```python
from build123d import *

# Parameters (mm, degrees)
SKETCH285_W     = 17
SKETCH285_H     = 21
PAD190_DEPTH    = 29
SKETCH281_W     = 13.1
SKETCH281_H     = 17
POCKET037_DEPTH = 25.7
SKETCH268_W     = 11.5
SKETCH268_H     = 1.2
SKETCH268_W_2   = 1.4
SKETCH268_H_2   = 2
POCKET039_DEPTH = 26.8
SKETCH271_R     = 0.6
POCKET041_DEPTH = 50
SKETCH278_W     = 0.6
SKETCH278_H     = 3
POCKET038_DEPTH = 2.5


with BuildPart() as part:
    # Sketch285 → Pad190 (new body)
    with BuildSketch(Plane.XZ):
        with Locations((1.5, 2)):
            Rectangle(SKETCH285_W, SKETCH285_H)
    extrude(amount=PAD190_DEPTH)

    # Sketch281 (on Face5 of Pad190) → Pocket037 (cut)
    with BuildSketch(Plane(origin=(0, 0, 0), x_dir=(1, 0, 0), z_dir=(0, 1, 0))):
        with Locations((2.05, -2)):
            Rectangle(SKETCH281_W, SKETCH281_H)
    extrude(amount=-POCKET037_DEPTH, mode=Mode.SUBTRACT)

    # Sketch268 (on Face4 of Pocket037) → Pocket039 (cut)
    with BuildSketch(Plane(origin=(0, 0, 0), x_dir=(1, 0, 0), z_dir=(0, 1, 0))):
        Rectangle(SKETCH268_W, SKETCH268_H)
        with Locations((9.3, -6)):
            Rectangle(SKETCH268_W_2, SKETCH268_H_2)
    extrude(amount=-POCKET039_DEPTH, mode=Mode.SUBTRACT)

    # Sketch271 (on Face6 of Pocket039) → Pocket041 (cut)
    with BuildSketch(Plane(origin=(0, 0, -8.5), x_dir=(1, 0, 0), z_dir=(0, 0, -1))):
        with Locations((0, 2)):
            Circle(SKETCH271_R)
    extrude(amount=-POCKET041_DEPTH, mode=Mode.SUBTRACT)

    # Sketch278 (on Face21 of Pocket041) → Pocket038 (cut)
    with BuildSketch(Plane(origin=(8.6, 0, 0), x_dir=(0, 0, 1), z_dir=(1, 0, 0))):
        with Locations((0, -9)):
            Rectangle(SKETCH278_W, SKETCH278_H)
    extrude(amount=-POCKET038_DEPTH, mode=Mode.SUBTRACT)


solid = part.part
```
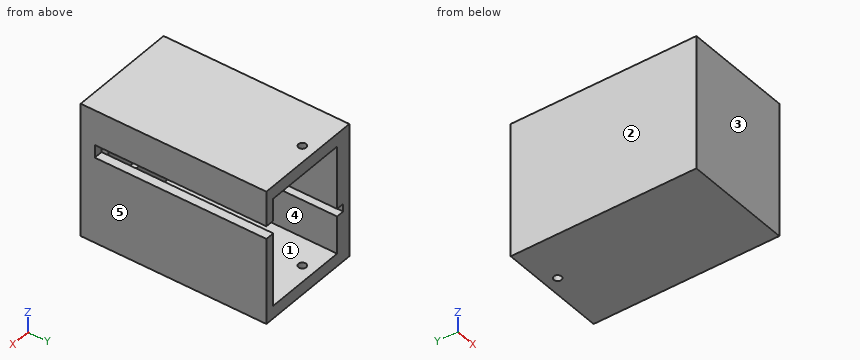
Read the model definition and answer for the solid it produces. Units are mm, in the model's axes. Face numbers are marked on the shaded views. A direction names the side the tool comes from. Coordinates: 2 decimals unless noted, no trailing zeros. Write each loop counter-clockwise with the first axis right and the second up, starting at its lowest first coordinate (ties: lowest second). Pieces come first, ordered by that corner, then holes. Notation, with made-up numbers: (19.25, -26) -> (35.25, -26) arc R16 cw to (35.25, -20) -> close; hole circle Ø9 at (72, 28). An arc over 180 degrees is marked (long way). Answer as a JSON object with one key per item and string values.
Q1. A tool of negligible diameter and unlimited length cuts with its end or side. For the marked faces 4 and 5, from which of +Z, -Z, +X, -X, +Y, -Y can it reach the whole face along a straight path? Write none if from no direction.
The answers:
{"face 4": "+Y", "face 5": "+Z, -Z, +X, +Y, -Y"}
Q2. The part is cut by section A-A on x = 0. Give the vertices of the cut face in (y, z).
The answers:
{"outline": "(-29, -8.5) -> (-2.6, -8.5) -> (-2.6, -6.5) -> (-25.7, -6.5) -> (-25.7, -0.6) -> (-26.8, -0.6) -> (-26.8, 0.6) -> (-25.7, 0.6) -> (-25.7, 10.5) -> (-2.6, 10.5) -> (-2.6, 12.5) -> (-29, 12.5) -> close; (-1.4, -8.5) -> (0, -8.5) -> (0, -6.5) -> (-1.4, -6.5) -> close; (-1.4, 10.5) -> (0, 10.5) -> (0, 12.5) -> (-1.4, 12.5) -> close"}
Q3. Determine the mould class of the marked faces 1, 2 and 3 for opening direction X: pulls with the +X half, pulls with the -X half, needs draft (parallel to the pull), parting line crosses it, or undercut.
The answers:
{"face 1": "undercut", "face 2": "pulls with the -X half", "face 3": "needs draft"}
Q4. The part is cut by section B-B on y = -2. Give the vertices of the cut face in (x, z).
The answers:
{"outline": "(-7, -8.5) -> (-0.6, -8.5) -> (-0.6, -6.5) -> (-4.5, -6.5) -> (-4.5, -0.6) -> (-5.75, -0.6) -> (-5.75, 0.6) -> (-4.5, 0.6) -> (-4.5, 10.5) -> (-0.6, 10.5) -> (-0.6, 12.5) -> (-7, 12.5) -> close; (0.6, -8.5) -> (10, -8.5) -> (10, 5) -> (8.6, 5) -> (8.6, -6.5) -> (0.6, -6.5) -> close; (0.6, 10.5) -> (8.6, 10.5) -> (8.6, 7) -> (10, 7) -> (10, 12.5) -> (0.6, 12.5) -> close"}
Q5. The part is cut by section D-D on z = -0.25. Give the vertices of the cut face in (x, y).
The answers:
{"outline": "(-7, -29) -> (10, -29) -> (10, 0) -> (8.6, 0) -> (8.6, -25.7) -> (5.75, -25.7) -> (5.75, -26.8) -> (-5.75, -26.8) -> (-5.75, 0) -> (-7, 0) -> close"}
Q6. The part is cut by section C-C on x = -4. Give the vertices of the cut face in (y, z).
The answers:
{"outline": "(-29, -8.5) -> (0, -8.5) -> (0, -6.5) -> (-25.7, -6.5) -> (-25.7, -0.6) -> (-26.8, -0.6) -> (-26.8, 0.6) -> (-25.7, 0.6) -> (-25.7, 10.5) -> (0, 10.5) -> (0, 12.5) -> (-29, 12.5) -> close"}
Q7. Flat-ended cylindrical pins translate along their axes: pin 1 Ø1.9 at (x, y) = (0, -2) entering from -Z; pin 2 Ø4 at (x, z) = (1, 3) entering from +Y. Find the tip coordinate at first contact, or state that the pin passes through.
The answers:
{"pin 1": "stops at z = -8.5", "pin 2": "stops at y = -25.7"}
Q8. Consider line 1 (X direction, y = -2, z = 11.55); line 2 (Z direction, x = 1.75, y = -25.75); line 3 (Z direction, x = 9, y = -8.75). Determine where each line is inside the solid, lowest interval first. Write a range as [from, to].
The answers:
{"line 1": "x = [-7, -0.6], [0.6, 10]", "line 2": "z = [-8.5, -0.6], [0.6, 12.5]", "line 3": "z = [-8.5, 5], [7, 12.5]"}
